from build123d import *

# Parameters (mm, degrees)
SKETCH1_R                       = 6
BOSS_EXTRUDE1_DEPTH             = 6
F_8_32_TAPPED_HOLE1_D           = 3.4544
F_8_32_TAPPED_HOLE1_DEPTH       = 5.1
F_8_32_TAPPED_HOLE1_CBORE_D     = 4.1656
F_8_32_TAPPED_HOLE1_CBORE_DEPTH = 4.2
F_8_32_TAPPED_HOLE1_TIP         = 1.037806461
CHAMFER1_SIZE                   = 0.1


with BuildPart() as part:
    # Sketch1 → Boss-Extrude1 (new body)
    with BuildSketch(Plane.XY):
        Circle(SKETCH1_R)
    extrude(amount=BOSS_EXTRUDE1_DEPTH)

    # #8-32 Tapped Hole1
    with Locations(Plane.XY.offset(6)):
        with Locations((0, 0)):
            CounterBoreHole(F_8_32_TAPPED_HOLE1_D / 2, F_8_32_TAPPED_HOLE1_CBORE_D / 2, F_8_32_TAPPED_HOLE1_CBORE_DEPTH, depth=F_8_32_TAPPED_HOLE1_DEPTH)
            with Locations((0, 0, -(F_8_32_TAPPED_HOLE1_DEPTH + F_8_32_TAPPED_HOLE1_TIP / 2))):  # 118° drill point
                Cone(0, F_8_32_TAPPED_HOLE1_D / 2, F_8_32_TAPPED_HOLE1_TIP, mode=Mode.SUBTRACT)

    # Chamfer1
    chamfer1_edges = [part.edges().sort_by_distance(p)[0] for p in [
        (-6, 0, 0),
        (-6, 0, 6),
    ]]
    chamfer(chamfer1_edges, length=CHAMFER1_SIZE)


solid = part.part
Here's how the part is built. I have some questions about the finished solid (model axes, mm). Give positions to 0.01 mm unless a question says otherwise; leave off trailing zeros. Order: outer loops, then holes, each group sorted by start corner. A loop starts at its lowest first (then second) coordinate and runs counter-clockwise, first axis right, second up. Notation, with made-up numbers: M -7.75,9 L 45.25,9 A23 ccw 45.25,24 Z; hole C -22,64 d3. An arc over 180 degrees is marked long. Answer as a JSON object with one key per item and string values. Group by question number.
1) Please list where these lines run through material, in increasing order: L1, parallel to Y at x = 0, z = 4.45; L2, parallel to Y at x = 0, z = 1.45; L3, parallel to X at y = 1.25, z = 4.45. Write a range as [from, to].
2) Suppose I cut it at C-C, the plane z = 4.35. Write out the boundary of the cut face in (x, y), plus the area to 3 significant figures.
3) We'd pull the mould along X, two halves only. Please class faces 1 (the cylindrical face through (0.225, 1.713, 1.344)), 2 (the flat face through (3, 0, 6)), 3 (the cylindrical face through (-6, 0, 3)), 4 (the cylindrical face through (1.987, 0.626, 3.929)): pulls with the +X half, pulls with the -X half, needs draft (parallel to the pull), parting line crosses it, or undercut.
4) I'm going to push a flat-ended pin straight in: pin 1 Ø5 at (x, y) = (4, -2.5) entering from -Z. Where does the tip first touch, or does it pass through?
5) Suppose I cut it at A-A, the plane y = 0. Write out the boundary of the cut face in (x, z).
Results found:
{
 "1": {"L1": "[-6, -2.08], [2.08, 6]", "L2": "[-6, -1.73], [1.73, 6]", "L3": "[-5.87, -1.67], [1.67, 5.87]"},
 "2": {"outline": "C 0,0 d12; hole C 0,0 d4.17", "area": "99.5 mm²"},
 "3": {"face 1": "undercut", "face 2": "needs draft", "face 3": "parting line crosses it", "face 4": "undercut"},
 "4": {"pin 1": "z = 0"},
 "5": {"outline": "M -6,0.1 L -5.9,0 L -0.23,0 L -1.73,0.9 L -1.73,1.8 L -2.08,1.8 L -2.08,6 L -5.9,6 L -6,5.9 Z; M 0.23,0 L 5.9,0 L 6,0.1 L 6,5.9 L 5.9,6 L 2.08,6 L 2.08,1.8 L 1.73,1.8 L 1.73,0.9 Z"}
}
